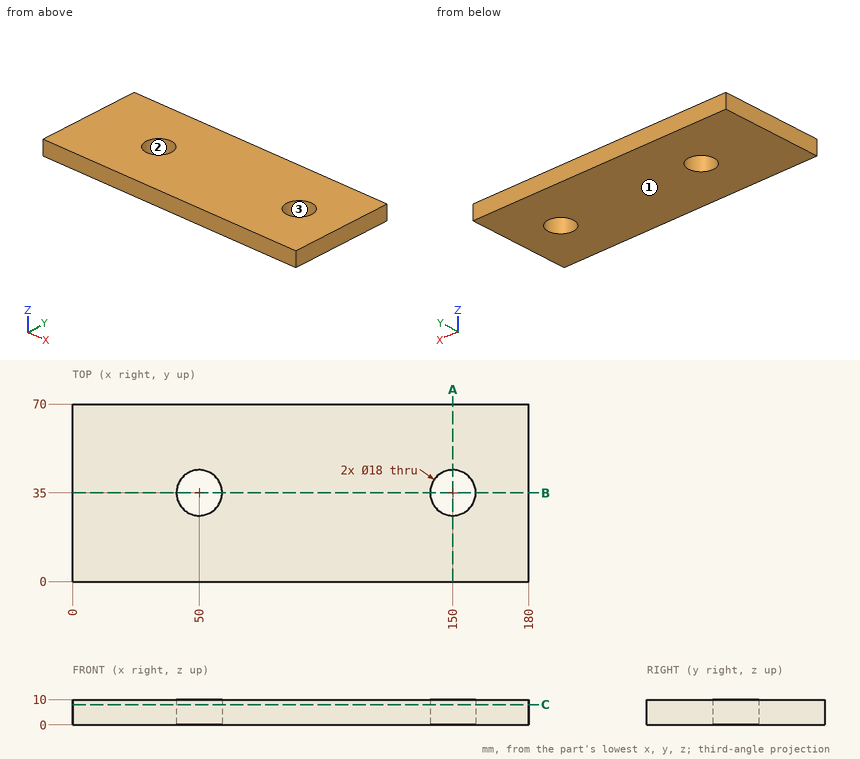
Check sheet for the drawn part. Datum: minimum x, y, z corner. Units: mm. Coordinates: 2 decimals unless noted, no trailing zeros. Order: outer loops, then holes, each group sorted by start corner. A loop starts at its lowest first (then second) coordinate and runs counter-clockwise, first axis right, second up. Notation, with made-up numbers: M -14,41 L 31,41 A19 ccw 31,67 Z; hole C -30,75 d2. An arc over 180 degrees is marked long. One line per item, written item: value. Start each with the question number.
Item 1: Mould release check, pull along Y, two halves, no side actions. Record for the marked faces 1, 2 and 3: released by +Y, released by -Y, zero draft, split by the parting line, or undercut.
Item 2: Sectioned sample at B-B (y = 35). Enter the section's corners in (x, z), then the cut area to 3 significant figures.
Item 3: Sectioned sample at C-C (z = 8). Enter the section's corners in (x, y).
Item 4: Scan lines: probe 1 along X at (y, z) = (35.5, 4.5); probe 2 along Y at (x, z) = (50, 2.5); probe 3 along X at (y, z) = (28, 7). Record each from-to range of solid material in increasing order.
Item 5: Sectioned sample at A-A (x = 150). Enter the section's corners in (y, z), then the cut area to 3 significant figures.
Conclusion:
1. face 1: zero draft
1. face 2: undercut
1. face 3: undercut
2. outline: M 0,0 L 41,0 L 41,10 L 0,10 Z; M 59,0 L 141,0 L 141,10 L 59,10 Z; M 159,0 L 180,0 L 180,10 L 159,10 Z
2. area: 1,440 mm^2
3. outline: M 0,0 L 180,0 L 180,70 L 0,70 Z; hole C 50,35 d18; hole C 150,35 d18
4. probe 1: x = 0 to 41.01, 58.99 to 141.01, 158.99 to 180
4. probe 2: y = 0 to 26, 44 to 70
4. probe 3: x = 0 to 44.34, 55.66 to 144.34, 155.66 to 180
5. outline: M 0,0 L 26,0 L 26,10 L 0,10 Z; M 44,0 L 70,0 L 70,10 L 44,10 Z
5. area: 520 mm^2
